The model under review builds one solid part; all positions refer to its coordinate system, in mm. A direction names the side the tool comes from. Coordinates: 2 decimals unless noted, no trailing zeros. Write each loop counter-clockwise with the first axis right and the second up, starting at its lowest first coordinate (ties: lowest second). Pieces come first, ordered by that corner, then holes. Notation, with made-up numbers: (-4.75, 83) - (21.25, 83) arc R27 cw to (21.25, 121) - close; hole circle Ø1 at (-6.5, 79.25). An arc over 180 degrees is marked (long way). Put each result on its own line as item: value.
from build123d import *

# Parameters (mm, degrees)
F1_DEPTH = 1066.8
F2_T     = -6.35


with BuildPart() as f1:
    # F0 (on Front) → F1 (new body, symmetric)
    with BuildSketch(Plane.XZ):
        with BuildLine():
            Line((168.275, 0), (-168.275, 0))
            Line((-168.275, 0), (-168.275, -200.025))
            ThreePointArc((-168.275, -200.025), (0, -368.3), (168.275, -200.025))
            Line((168.275, -200.025), (168.275, 0))
        make_face()
    extrude(amount=F1_DEPTH, both=True)

    # F2
    f2_openings = [f1.faces().sort_by_distance(p)[0] for p in [
        (0, 0, 0),
    ]]
    offset(amount=F2_T, openings=f2_openings)


solid = f1.part
1. Consider section D-D on z = -309. State the section outline as (x, y) points, plus the area to 3 significant figures.
Determined:
outline: (-128.22, -1066.8) - (128.22, -1066.8) - (128.22, 1066.8) - (-128.22, 1066.8) - close; hole (-119.77, -1060.45) - (119.77, -1060.45) - (119.77, 1060.45) - (-119.77, 1060.45) - close
area: 39,100 mm^2
2. Consider section A-A on z = -65.5. State the section outline as (x, y) points (3 decimals).
Determined:
outline: (-168.275, -1066.8) - (168.275, -1066.8) - (168.275, 1066.8) - (-168.275, 1066.8) - close; hole (-161.925, -1060.45) - (161.925, -1060.45) - (161.925, 1060.45) - (-161.925, 1060.45) - close
3. The part is to be moulded in two halves that separate along Y. For faces 3 (the flat face through (-2, -1060.45, -178)), 4 (the flat face through (-2, -1066.8, -182)), 5 (the flat face through (-168.275, -15, -99)), say which applies: +Y half, -Y half, draft (parallel to the pull), parting line (faces both ways), or undercut.
Determined:
face 3: undercut
face 4: -Y half
face 5: draft
4. Machinability: for faces 1 (the flat face through (161.925, -15, -101)), 2 (the flat face through (-2, 1066.8, -182)), which of the approach directions +Z, -Z, +X, -X, +Y, -Y give a long, thin tool a straight path to every point of the face, cutting with its end or side? Answer none if there is none.
Determined:
face 1: +Z
face 2: +Z, -Z, +X, -X, +Y
5. For pin 1 Ø6 at (x, y) = (-51, -455.5) entering from -Z; pin 2 Ø5 at (y, z) = (278, -270.5) entering from -X; pin 3 Ø10 at (x, y) = (90, 57.5) entering from -Z, all flat-tipped, find the tip position at first contact; note any pin that passes through.
Determined:
pin 1: stops at z = -361.31
pin 2: stops at x = -153.93
pin 3: stops at z = -345.25
6. Consider section B-B on x = 0. State the section outline as (y, z) points, plus the area to 3 significant figures.
Determined:
outline: (-1066.8, -368.3) - (1066.8, -368.3) - (1066.8, 0) - (1060.45, 0) - (1060.45, -361.95) - (-1060.45, -361.95) - (-1060.45, 0) - (-1066.8, 0) - close
area: 18,100 mm^2
7. To check wall thickness, follow probe 1 along X at (y, z) = (908.5, -143) (3 decimals); probe 2 along Y at (x, z) = (-39, -112.5); probe 3 along X at (y, z) = (410, -253.5). State the ranges of each line that lie inside material, in increasing order.
Determined:
probe 1: x = -168.275 to -161.925, 161.925 to 168.275
probe 2: y = -1066.8 to -1060.45, 1060.45 to 1066.8
probe 3: x = -159.55 to -152.84, 152.84 to 159.55
8. Consider section C-C on y = -297. State the section outline as (x, z) points (3 decimals), plus the area to 3 significant figures.
Determined:
outline: (-168.275, -200.025) arc R168.275 ccw to (168.275, -200.025) - (168.275, 0) - (161.925, 0) - (161.925, -200.025) arc R161.925 cw to (-161.925, -200.025) - (-161.925, 0) - (-168.275, 0) - close
area: 5,830 mm^2
